from build123d import *

# Parameters (mm, degrees)
F1_DEPTH       = 20
F3_DEPTH       = 17.4
F4_D           = 5
F4_DEPTH       = 5.001
F5_D           = 5
F7_D           = 3.3
F7_CSINK_D     = 6.72
F7_CSINK_ANGLE = 90


with BuildPart() as f1:
    # F0 (on Right) → F1 (new body)
    with BuildSketch(Plane.YZ):
        Polygon((-2.3540243498, -11.660939306), (-2.3540243498, 8.339060694), (-20.3540243498, 8.339060694), (-20.3540243498, 3.339060694), (-7.3540243498, 3.339060694), (-7.3540243498, -6.660939306), (-20.3540243498, -6.660939306), (-20.3540243498, -11.660939306), align=None)
    extrude(amount=F1_DEPTH)

    # F2 (on face) → F3 (cut, symmetric)
    with BuildSketch(Plane.XY.offset(-6.660939306)):
        with BuildLine():
            ThreePointArc((10, -20.3540243498), (6.8012442082, -19.4302396116), (4.5874756769, -16.9433448113))
            Line((4.5874756769, -16.9433448113), (0, -7.3540243498))
            Line((0, -7.3540243498), (0, -20.3540243498))
            Line((0, -20.3540243498), (10, -20.3540243498))
        make_face()
        with BuildLine():
            ThreePointArc((15.4125243231, -16.9433448113), (13.1987557918, -19.4302396116), (10, -20.3540243498))
            Line((10, -20.3540243498), (20, -20.3540243498))
            Line((20, -20.3540243498), (20, -7.3540243498))
            Line((20, -7.3540243498), (15.4125243231, -16.9433448113))
        make_face()
    extrude(amount=F3_DEPTH, both=True, mode=Mode.SUBTRACT)

    # F4 (through all, one way)
    with BuildSketch(Plane.XY.offset(-6.660939306)):
        with Locations((10, -14.3540243498)):
            Circle(F4_D / 2)
    extrude(amount=-F4_DEPTH, mode=Mode.SUBTRACT)

    # F5 (through all)
    with Locations(Plane(origin=(0, 0, -6.660939306), x_dir=(1, 0, 0), z_dir=(0, 0, -1))):
        with Locations((10, 14.3540243498)):
            Hole(F5_D / 2)

    # F7 (through all)
    with Locations(Plane.XZ.offset(7.3540243498)):
        with Locations((5, -1.751396223), (15, -1.660939306)):
            CounterSinkHole(F7_D / 2, F7_CSINK_D / 2, counter_sink_angle=F7_CSINK_ANGLE)


solid = f1.part
The listing builds one solid part. Answer for the finished solid, in the listing's coordinates (mm). A direction names the side the tool comes from. Give positions to 0.01 mm unless a question says otherwise; leave off trailing zeros. Write each loop counter-clockwise with the first axis right and the second up, starting at its lowest first coordinate (ties: lowest second). Pieces come first, ordered by that corner, then holes.
Item 1: Section B-B, the plane x = 9.5 is taken. Write down the section's boundary in (y, z).
Item 2: Section A-A, the plane y = -9.25 is taken. Write down the section's boundary in (x, z).
Item 3: Section D-D, the plane x = 5 is taken. Write down the section's boundary in (y, z).
Item 4: Flat-ended cylindrical pins translate along their axes: P1, Ø6, axis at x = 13.5, z = 5.5, coming from the -Y side; P2, Ø4, axis at x = 6.5, z = -7.5, coming from the -Y side; P3, Ø4.5, axis at x = 15, z = -1.66, coming from the -Y side. Find the tip coordinate at first contact, or state that the pin passes through.
Item 5: Determine the mould class of faces 1 (the flat face through (10, -11, -6.661)), 2 (the flat face through (0, -5, -2)), 3 (the flat face through (10, -9, 8.339)) for opening direction Z: released by +Z, released by -Z, zero draft, split by the parting line, or undercut.
Item 6: Find the intervals of material crossed by line 1 along Y through (x, z) = (10, 6.25); line 2 along Z through (x, y) = (6.5, -12.25); line 3 along Z through (x, y) = (5, -3.1), in increasing order.
Item 7: Which of the six approach directions +Z, -Z, +X, -X, +Y, -Y give full straight-line access (tool end or side, diameter ignored) to faces 4 (the flat face through (10, -11, 3.339)), 5 (the flat face through (2.33, -12.22, -9.13))?
Item 8: Section C-C, the plane z = 5 is taken. Write down the section's boundary in (x, y).
Completed:
1. outline: (-20.33, -11.66) - (-16.8, -11.66) - (-16.8, -6.66) - (-20.33, -6.66) - close; (-20.33, 3.34) - (-16.8, 3.34) - (-16.8, 8.34) - (-20.33, 8.34) - close; (-11.9, -11.66) - (-2.35, -11.66) - (-2.35, 8.34) - (-11.9, 8.34) - (-11.9, 3.34) - (-7.35, 3.34) - (-7.35, -6.66) - (-11.9, -6.66) - close
2. outline: (0.91, -11.66) - (19.09, -11.66) - (19.09, -6.66) - (0.91, -6.66) - close; (0.91, 3.34) - (19.09, 3.34) - (19.09, 8.34) - (0.91, 8.34) - close
3. outline: (-17.67, -11.66) - (-2.35, -11.66) - (-2.35, -3.4) - (-5.64, -3.4) - (-7.35, -5.11) - (-7.35, -6.66) - (-17.67, -6.66) - close; (-17.67, 3.34) - (-7.35, 3.34) - (-7.35, 1.61) - (-5.64, -0.1) - (-2.35, -0.1) - (-2.35, 8.34) - (-17.67, 8.34) - close
4. P1: stops at y = -20.33
4. P2: stops at y = -20.16
4. P3: stops at y = -6.24
5. face 1: undercut
5. face 2: zero draft
5. face 3: released by +Z
6. line 1: y = -20.35 to -16.85, -11.85 to -2.35
6. line 2: z = -11.66 to -6.66, 3.34 to 8.34
6. line 3: z = -11.66 to -3.4, -0.1 to 8.34
7. face 4: +X, -X, -Y
7. face 5: +Z, -Z, -X, -Y
8. outline: (0, -7.35) - (4.59, -16.94) arc R6 ccw to (15.41, -16.94) - (20, -7.35) - (20, -2.35) - (0, -2.35) - close; hole circle Ø5 at (10, -14.35)
